Verification items for the finished model (mm, model axes). A direction names the side the tool comes from. Coordinates: 2 decimals unless noted, no trailing zeros. Loops run counter-clockwise (first coordinate to the right, second up) from the corner with the lowest first, then second, coordinate; pieces in that order, holes last.
Q1. Go/stop test with flat-tipped pins: P1, Ø1.5, axis at x = 42.5, y = 48, coming from the +Z side; P2, Ø1, axis at x = 59.5, y = 9.5, coming from the +Z side; P3, Ø1.8, axis at x = 43.5, y = 46, coming from the -Z side; P4, Ø6.5, axis at x = -9.5, y = 48.7, coming from the -Z side. Record where each tip stops, or that it passes through.
Q2. Sectioned sample at A-A (y = 29.35). Enter the section's corners in (x, z).
Q3. Sectioned sample at B-B (z = -46.5). Enter the section's corners in (x, y), then the cut area to 3 significant figures.
Q4. Sectioned sample at C-C (x = 68). Enter the section's corners in (y, z).
Q5. Material ranges on probe 1 along X at (y, z) = (19.5, -34); probe 2 along X at (y, z) = (44.5, -65.5), recorded low to high.
Q6. Access from +Z, -Z, +X, -X, +Y, -Y to the whole of each face (thin tool, end or side, straight path). Record for faces 5 (the face through (57.8, 0.86, -50.01)), 6 (the face through (23, 5, -7)), 7 (the face through (8, 29, -26)), 8 (the face through (43.6, 43.6, -57)), 9 (the face through (0.9, 57.84, -50.01)).
Q7. Mould release check, pull along X, two halves, no side actions. Record for faces 1 (the face through (44.044, 46.115, -55.028)), 2 (the face through (29, 50.7, -26)), 3 (the face through (-16.147, 57.798, -3.549)), 4 (the face through (29, 17, -86)): +X half, -X half, draft (parallel to the pull), parting line (faces both ways), or undercut.
```python
from build123d import *

# Parameters (mm, degrees)
CROQUIS1_W              = 58.7
CROQUIS1_H              = 58.7
SALIENTE_EXTRUIR1_DEPTH = 86
CROQUIS2_W              = 42.7
CROQUIS2_H              = 42.7
CORTAR_EXTRUIR1_DEPTH   = 53
CROQUIS3_R              = 18.5
CORTAR_EXTRUIR2_DEPTH   = 30
CROQUIS4_R              = 11.5
CORTAR_EXTRUIR3_DEPTH   = 118.389863276
CROQUIS5_R              = 1.5
CORTAR_EXTRUIR4_DEPTH   = 118.389863276
MATRIZC1_COUNT          = 4
CORTAR_EXTRUIR5_DEPTH   = 5
CROQUIS7_W              = 92.702698273
CROQUIS7_H              = 58.7
CROQUIS7_R              = 2.5
CROQUIS7_W_2            = 42.7
CROQUIS7_H_2            = 42.7
SALIENTE_EXTRUIR2_DEPTH = 10
CROQUIS9_W              = 12.7
CROQUIS9_H              = 8
CORTAR_EXTRUIR7_DEPTH   = 15
REDONDEO1_R             = 3
CORTAR_EXTRUIR8_DEPTH   = 29
CROQUIS11_R             = 1.5
CORTAR_EXTRUIR9_DEPTH   = 4


with BuildPart() as part:
    # Croquis1 → Saliente-Extruir1 (new body)
    with BuildSketch(Plane.XY):
        with Locations((29.35, 29.35)):
            Rectangle(CROQUIS1_W, CROQUIS1_H)
    extrude(amount=-SALIENTE_EXTRUIR1_DEPTH)

    # Croquis2 → Cortar-Extruir1 (cut)
    with BuildSketch(Plane.XY):
        with Locations((29.35, 29.35)):
            Rectangle(CROQUIS2_W, CROQUIS2_H)
    extrude(amount=-CORTAR_EXTRUIR1_DEPTH, mode=Mode.SUBTRACT)

    # Croquis3 → Cortar-Extruir2 (cut)
    with BuildSketch(Plane.XY.offset(-53)):
        with Locations((29.35, 29.35)):
            Circle(CROQUIS3_R)
    extrude(amount=-CORTAR_EXTRUIR2_DEPTH, mode=Mode.SUBTRACT)

    # Croquis4 → Cortar-Extruir3 (cut, through all)
    with BuildSketch(Plane.XY.offset(-83)):
        with Locations((29.35, 29.35)):
            Circle(CROQUIS4_R)
    extrude(amount=-CORTAR_EXTRUIR3_DEPTH, mode=Mode.SUBTRACT)

    # Croquis5 → Cortar-Extruir4 (cut, through all)
    with BuildSketch(Plane.XY.offset(-83)):
        with Locations((39.249494937, 39.249494937)):
            Circle(CROQUIS5_R)
    cortar_extruir4 = extrude(amount=-CORTAR_EXTRUIR4_DEPTH, mode=Mode.SUBTRACT)

    # MatrizC1: Cortar-Extruir4 ×4 about axis
    matrizc1_axis = Axis((29.35, 29.35, 0), (0, 0, 1))
    for i in range(1, MATRIZC1_COUNT):
        add(cortar_extruir4.rotate(matrizc1_axis, i * 360 / MATRIZC1_COUNT), mode=Mode.SUBTRACT)

    # Croquis6 → Cortar-Extruir5 (cut)
    with BuildSketch(Plane(origin=(0, 0, -86), x_dir=(-1, 0, 0), z_dir=(0, 0, -1))):
        with BuildLine():
            ThreePointArc((-29.35, 53.35), (-30.35, 52.35), (-29.35, 51.35))
            Line((-29.35, 51.35), (-29.35, 53.35))
        make_face()
        with BuildLine():
            Line((-29.35, 53.35), (-29.35, 51.35))
            ThreePointArc((-29.35, 51.35), (-28.642893219, 51.642893219), (-28.35, 52.35))
            ThreePointArc((-28.35, 52.35), (-28.642893219, 53.057106781), (-29.35, 53.35))
        make_face()
        with BuildLine():
            ThreePointArc((-29.35, 46.6), (-30.35, 45.6), (-29.35, 44.6))
            Line((-29.35, 44.6), (-29.35, 46.6))
        make_face()
        with BuildLine():
            Line((-29.35, 46.6), (-29.35, 44.6))
            ThreePointArc((-29.35, 44.6), (-28.642893219, 44.892893219), (-28.35, 45.6))
            ThreePointArc((-28.35, 45.6), (-28.642893219, 46.307106781), (-29.35, 46.6))
        make_face()
        with BuildLine():
            ThreePointArc((-29.35, 14.1), (-30.35, 13.1), (-29.35, 12.1))
            Line((-29.35, 12.1), (-29.35, 14.1))
        make_face()
        with BuildLine():
            Line((-29.35, 14.1), (-29.35, 12.1))
            ThreePointArc((-29.35, 12.1), (-28.642893219, 12.392893219), (-28.35, 13.1))
            ThreePointArc((-28.35, 13.1), (-28.642893219, 13.807106781), (-29.35, 14.1))
        make_face()
        with BuildLine():
            ThreePointArc((-29.35, 7.35), (-30.35, 6.35), (-29.35, 5.35))
            Line((-29.35, 5.35), (-29.35, 7.35))
        make_face()
        with BuildLine():
            Line((-29.35, 7.35), (-29.35, 5.35))
            ThreePointArc((-29.35, 5.35), (-28.642893219, 5.642893219), (-28.35, 6.35))
            ThreePointArc((-28.35, 6.35), (-28.642893219, 7.057106781), (-29.35, 7.35))
        make_face()
    extrude(amount=-CORTAR_EXTRUIR5_DEPTH, mode=Mode.SUBTRACT)

    # Croquis7 → Saliente-Extruir2 (add)
    with BuildSketch(Plane.XY):
        with Locations((29.348650864, 29.35)):
            Rectangle(CROQUIS7_W, CROQUIS7_H)
        with Locations((-9.502698273, 48.7)):
            Circle(CROQUIS7_R, mode=Mode.SUBTRACT)
        with Locations((68.2, 48.7)):
            Circle(CROQUIS7_R, mode=Mode.SUBTRACT)
        with Locations((-9.502698273, 8.7)):
            Circle(CROQUIS7_R, mode=Mode.SUBTRACT)
        with Locations((68.2, 8.7)):
            Circle(CROQUIS7_R, mode=Mode.SUBTRACT)
        with Locations((29.35, 29.35)):
            Rectangle(CROQUIS7_W_2, CROQUIS7_H_2, mode=Mode.SUBTRACT)
    extrude(amount=-SALIENTE_EXTRUIR2_DEPTH)

    # Croquis9 → Cortar-Extruir7 (cut)
    with BuildSketch(Plane.XY):
        with Locations((29.35, 4)):
            Rectangle(CROQUIS9_W, CROQUIS9_H)
    extrude(amount=-CORTAR_EXTRUIR7_DEPTH, mode=Mode.SUBTRACT)

    # Redondeo1
    redondeo1_edges = [part.edges().sort_by_distance(p)[0] for p in [
        (0, 0, -48),
        (23, 0, -7.5),
        (29.35, 0, -15),
        (35.7, 0, -7.5),
        (-8.501349137, 58.7, -10),
        (-17.002698273, 58.7, -5),
        (-8.501349137, 0, -10),
        (0, 29.35, -10),
        (58.7, 29.35, -10),
        (-17.002698273, 29.35, -10),
        (0, 58.7, -48),
        (-17.002698273, 0, -5),
        (67.2, 58.7, -10),
        (75.7, 29.35, -10),
        (58.7, 58.7, -48),
        (75.7, 58.7, -5),
        (67.2, 0, -10),
        (75.7, 0, -5),
        (58.7, 0, -48),
    ]]
    fillet(redondeo1_edges, radius=REDONDEO1_R)

    # Croquis10 → Cortar-Extruir8 (cut)
    with BuildSketch(Plane(origin=(0, 0, -86), x_dir=(-1, 0, 0), z_dir=(0, 0, -1))):
        with BuildLine():
            ThreePointArc((-41.85, 44.85), (-46.971320344, 46.971320344), (-44.85, 41.85))
            Line((-44.85, 41.85), (-44.85, 44.85))
            Line((-44.85, 44.85), (-41.85, 44.85))
        make_face()
        with BuildLine():
            Line((-44.85, 44.85), (-44.85, 41.85))
            ThreePointArc((-44.85, 41.85), (-42.728679656, 42.728679656), (-41.85, 44.85))
            Line((-41.85, 44.85), (-44.85, 44.85))
        make_face()
        with BuildLine():
            ThreePointArc((-16.85, 44.85), (-15.971320344, 42.728679656), (-13.85, 41.85))
            Line((-13.85, 41.85), (-13.85, 44.85))
            Line((-13.85, 44.85), (-16.85, 44.85))
        make_face()
        with BuildLine():
            Line((-13.85, 44.85), (-13.85, 41.85))
            ThreePointArc((-13.85, 41.85), (-11.728679656, 42.728679656), (-10.85, 44.85))
            ThreePointArc((-10.85, 44.85), (-13.85, 47.85), (-16.85, 44.85))
            Line((-16.85, 44.85), (-13.85, 44.85))
        make_face()
        with BuildLine():
            ThreePointArc((-13.85, 16.85), (-15.971320344, 15.971320344), (-16.85, 13.85))
            Line((-16.85, 13.85), (-13.85, 13.85))
            Line((-13.85, 13.85), (-13.85, 16.85))
        make_face()
        with BuildLine():
            Line((-13.85, 13.85), (-16.85, 13.85))
            ThreePointArc((-16.85, 13.85), (-13.85, 10.85), (-10.85, 13.85))
            ThreePointArc((-10.85, 13.85), (-11.728679656, 15.971320344), (-13.85, 16.85))
            Line((-13.85, 16.85), (-13.85, 13.85))
        make_face()
        with BuildLine():
            Line((-44.85, 16.85), (-44.85, 13.85))
            Line((-44.85, 13.85), (-41.85, 13.85))
            ThreePointArc((-41.85, 13.85), (-42.728679656, 15.971320344), (-44.85, 16.85))
        make_face()
        with BuildLine():
            Line((-41.85, 13.85), (-44.85, 13.85))
            Line((-44.85, 13.85), (-44.85, 16.85))
            ThreePointArc((-44.85, 16.85), (-46.971320344, 11.728679656), (-41.85, 13.85))
        make_face()
    extrude(amount=-CORTAR_EXTRUIR8_DEPTH, mode=Mode.SUBTRACT)

    # Croquis11 → Cortar-Extruir9 (cut)
    with BuildSketch(Plane(origin=(0, 0, -57), x_dir=(-1, 0, 0), z_dir=(0, 0, -1))):
        with Locations((-44.85, 44.85)):
            Circle(CROQUIS11_R)
        with Locations((-13.85, 44.85)):
            Circle(CROQUIS11_R)
        with Locations((-13.85, 13.85)):
            Circle(CROQUIS11_R)
        with Locations((-44.85, 13.85)):
            Circle(CROQUIS11_R)
    extrude(amount=-CORTAR_EXTRUIR9_DEPTH, mode=Mode.SUBTRACT)


solid = part.part
```
Geometry check:
1. P1: stops at z = -53
1. P2: stops at z = 0
1. P3: stops at z = -57
1. P4: stops at z = -10
2. outline: (-17, -7) arc R3 ccw to (-14, -10) - (-3, -10) arc R3 cw to (0, -13) - (0, -86) - (17.85, -86) - (17.85, -83) - (10.85, -83) - (10.85, -53) - (8, -53) - (8, 0) - (-17, 0) - close; (40.85, -86) - (58.7, -86) - (58.7, -13) arc R3 cw to (61.7, -10) - (72.7, -10) arc R3 ccw to (75.7, -7) - (75.7, 0) - (50.7, 0) - (50.7, -53) - (47.85, -53) - (47.85, -83) - (40.85, -83) - close
3. outline: (0, 3) arc R3 ccw to (3, 0) - (55.7, 0) arc R3 ccw to (58.7, 3) - (58.7, 55.7) arc R3 ccw to (55.7, 58.7) - (3, 58.7) arc R3 ccw to (0, 55.7) - close; hole (8, 8) - (50.7, 8) - (50.7, 50.7) - (8, 50.7) - close
3. area: 1,610 mm2
4. outline: (0, -7) arc R3 ccw to (3, -10) - (6.21, -10) - (6.21, 0) - (0, 0) - close; (11.19, -10) - (46.21, -10) - (46.21, 0) - (11.19, 0) - close; (51.19, -10) - (55.7, -10) arc R3 ccw to (58.7, -7) - (58.7, 0) - (51.19, 0) - close
5. probe 1: x = 0 to 8, 50.7 to 58.7
5. probe 2: x = 0 to 10.87, 16.83 to 18.73, 39.97 to 41.87, 47.83 to 58.7
6. face 5: -Z, +X, -Y
6. face 6: +Z, -Y
6. face 7: +Z
6. face 8: -Z
6. face 9: -Z, -X, +Y
7. face 1: undercut
7. face 2: undercut
7. face 3: -X half
7. face 4: draft
